```python
from build123d import *

# Parameters (mm, degrees)
F0_R     = 2
F0_W     = 0.8
F0_H     = 34
F1_DEPTH = 0.8
F2_W     = 0.8
F2_H     = 34
F3_DEPTH = 12.7
F5_R     = 6.35
F6_D     = 4
F7_R     = 0.5


with BuildPart() as f1:
    # F0 (on Top) → F1 (new body)
    with BuildSketch(Plane.XY):
        Polygon((11.3, 17), (11.3, 18.4), (-11.3, 18.4), (-11.3, 17), (-11.3, -17), (-11.3, -18.4), (11.3, -18.4), (11.3, -17), align=None)
        with Locations((-6.35, -12.7)):
            Circle(F0_R, mode=Mode.SUBTRACT)
        with Locations((6.35, -12.7)):
            Circle(F0_R, mode=Mode.SUBTRACT)
        with Locations((-6.35, 0)):
            Circle(F0_R, mode=Mode.SUBTRACT)
        with Locations((-6.35, 12.7)):
            Circle(F0_R, mode=Mode.SUBTRACT)
        with Locations((6.35, 0)):
            Circle(F0_R, mode=Mode.SUBTRACT)
        with Locations((6.35, 12.7)):
            Circle(F0_R, mode=Mode.SUBTRACT)
        with Locations((11.7, 0)):
            Rectangle(F0_W, F0_H)
        with Locations((-11.7, 0)):
            Rectangle(F0_W, F0_H)
    extrude(amount=F1_DEPTH)

    # F2 (on face) → F3 (join)
    with BuildSketch(Plane.XY.offset(0.8)):
        with Locations((-11.7, 0)):
            Rectangle(F2_W, F2_H)
        with Locations((11.7, 0)):
            Rectangle(F2_W, F2_H)
    extrude(amount=F3_DEPTH)

    # F5
    f5_edges = [f1.edges().sort_by_distance(p)[0] for p in [
        (11.7, 17, 13.5),
        (-11.7, 17, 13.5),
        (11.7, -17, 13.5),
        (-11.7, -17, 13.5),
    ]]
    fillet(f5_edges, radius=F5_R)

    # F6 (through all)
    with Locations(Plane.YZ.offset(12.1)):
        with Locations((-12.7, 7.15), (0, 7.15), (12.7, 7.15)):
            Hole(F6_D / 2)

    # F7
    f7_edges = [f1.edges().sort_by_distance(p)[0] for p in [
        (12.1, 0, 0),
        (-12.1, 0, 0),
    ]]
    fillet(f7_edges, radius=F7_R)


solid = f1.part
```
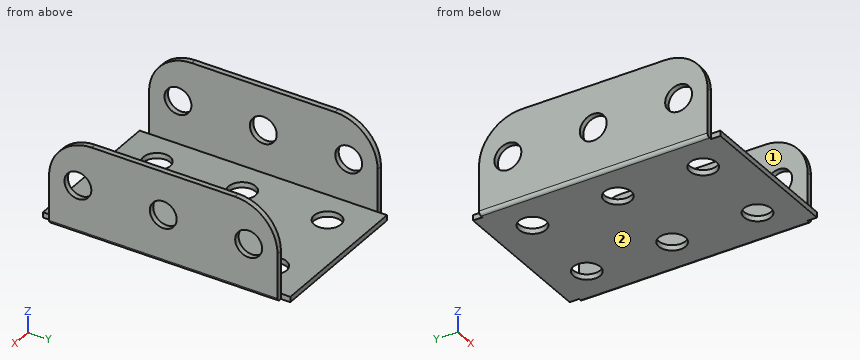
Work out the finished part from the listing and answer in its coordinate system (mm). Face numbers are marked on the shaded views. A direction names the side the tool comes from. Give positions to 0.01 mm unless a question says otherwise; leave off trailing zeros. Order: outer loops, then holes, each group sorted by start corner. A loop starts at its lowest first (then second) coordinate and runs counter-clockwise, first axis right, second up.
1. Section A-A, the plane z = 8 is taken. Give the number of separate pieces and of enclosed holes in the cut face, and give its area (3 significant figures).
Result sheet:
separate pieces: 8
enclosed holes: 0
area: 36.8 mm2
2. Section C-C, the plane x = 6.35 is taken. Determine the outline of the cut face in (y, z), and give its area (3 significant figures).
Result sheet:
outline: (-18.4, 0) - (-14.7, 0) - (-14.7, 0.8) - (-18.4, 0.8) - close; (-10.7, 0) - (-2, 0) - (-2, 0.8) - (-10.7, 0.8) - close; (2, 0) - (10.7, 0) - (10.7, 0.8) - (2, 0.8) - close; (14.7, 0) - (18.4, 0) - (18.4, 0.8) - (14.7, 0.8) - close
area: 19.8 mm2
3. Straight lines are drawn through the part: L1, parallel to Y at x = -6.35, z = 0.65; L2, parallel to X at y = -5, z = 10; L3, parallel to Z at x = 2.25, y = -4.5. For each, find the intervals that lie inside material, in ascending order.
Result sheet:
L1: y = -18.4 to -14.7, -10.7 to -2, 2 to 10.7, 14.7 to 18.4
L2: x = -12.1 to -11.3, 11.3 to 12.1
L3: z = 0 to 0.8
4. For the marked faces 1 and 2, determine the directions among +Z, -Z, +X, -X, +Y, -Y from which every point of the face is accessible in a straight line to the end or side of a thin tool.
Result sheet:
face 1: +Z, +Y, -Y
face 2: -Z, +X, -X, +Y, -Y
5. Each of these flat-tipped pins is pushed along its axis until it touches: P1, Ø0.9, axis at y = -18, z = 0.5, coming from the -X side; P2, Ø8, axis at x = -5, y = -1.5, coming from the +Z side; P3, Ø0.6, axis at x = -11.5, z = 3.5, coming from the +Y side. Where does it stop, or does it pass through?
Result sheet:
P1: stops at x = -11.3
P2: stops at z = 0.8
P3: stops at y = 17
6. Section D-D, the plane z = 4 is taken. Determine the outline of the cut face in (x, y), and give its area (3 significant figures).
Result sheet:
outline: (-12.1, -17) - (-11.3, -17) - (-11.3, 17) - (-12.1, 17) - close; (11.3, -17) - (12.1, -17) - (12.1, 17) - (11.3, 17) - close
area: 54.4 mm2
7. Section B-B, the plane y = -12.7 is taken. Determine the outline of the cut face in (x, z), and give its area (3 significant figures).
Result sheet:
outline: (-12.1, 0.5) arc R0.5 ccw to (-11.6, 0) - (-8.35, 0) - (-8.35, 0.8) - (-11.3, 0.8) - (-11.3, 5.15) - (-12.1, 5.15) - close; (-12.1, 9.15) - (-11.3, 9.15) - (-11.3, 13.16) - (-12.1, 13.16) - close; (-4.35, 0) - (4.35, 0) - (4.35, 0.8) - (-4.35, 0.8) - close; (8.35, 0) - (11.6, 0) arc R0.5 ccw to (12.1, 0.5) - (12.1, 5.15) - (11.3, 5.15) - (11.3, 0.8) - (8.35, 0.8) - close; (11.3, 9.15) - (12.1, 9.15) - (12.1, 13.16) - (11.3, 13.16) - close
area: 26.2 mm2
